from build123d import *

# Parameters (mm, degrees)
CHANFREIN1_SIZE         = 0.2
CONG_1_R                = 0.5
EMPREINTE_POUR_CL_DEPTH = 2.5


with BuildPart() as part:
    # Esquisse1 → Base-Révolution (revolve)
    with BuildSketch(Plane.XY, mode=Mode.PRIVATE) as base_r_volution_sk:
        Polygon((-2.5, 0), (-2.5, 2.25), (0, 2.25), (0, 1.25), (10, 1.25), (10, 0), align=None)
    revolve(base_r_volution_sk.sketch.rotate(Axis((-28.982684825, 0, 0), (1, 0, 0)), 90), axis=Axis((-28.982684825, 0, 0), (1, 0, 0)))

    # Chanfrein1
    chanfrein1_edges = [part.edges().sort_by_distance(p)[0] for p in [
        (10, 0, -1.25),
    ]]
    chamfer(chanfrein1_edges, length=CHANFREIN1_SIZE)

    # Congé1
    cong_1_edges = [part.edges().sort_by_distance(p)[0] for p in [
        (-2.5, 0, -2.25),
    ]]
    fillet(cong_1_edges, radius=CONG_1_R)

    # Esquisse2 → Empreinte pour clé (cut)
    with BuildSketch(Plane.ZY.offset(2.5)):
        Polygon((0.577350269, -1), (-0.577350269, -1), (-1.154700538, 0), (-0.577350269, 1), (0.577350269, 1), (1.154700538, 0), align=None)
    extrude(amount=-EMPREINTE_POUR_CL_DEPTH, mode=Mode.SUBTRACT)


solid = part.part
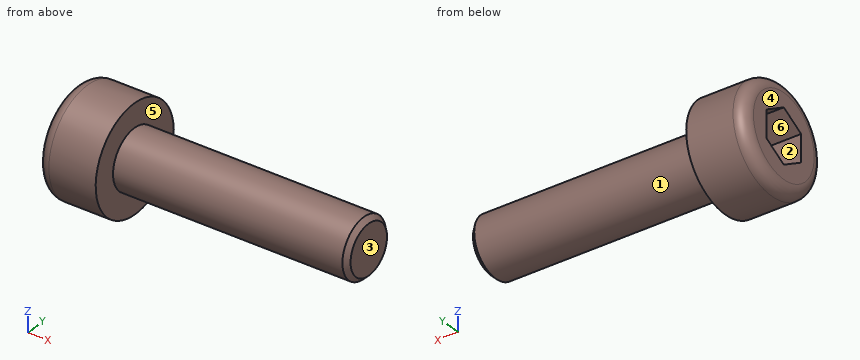
Work out the finished part from the listing and answer in its coordinate system (mm). Face numbers are marked on the shaded views. A direction names the side the tool comes from. Coordinates: 2 decimals unless noted, no trailing zeros. Write each loop counter-clockwise with the first axis right and the second up, starting at its lowest first coordinate (ties: lowest second). Pieces come first, ordered by that corner, then holes. Notation, with made-up numbers: (25.25, 64) - (56.25, 64) arc R30 cw to (56.25, 99) - close; hole circle Ø6 at (-15.75, 81.25). An arc over 180 degrees is marked (long way). One line per question, with ' | ' between items.
1) Consider probe 1 along X at (y, z) = (1, -1.2); probe 2 along X at (y, z) = (-0.05, 0.5); probe 3 along Y at (x, z) = (-0.75, 1.5). Determine where each line is inside the solid, lowest interval first. Write a range as [from, to].
Checks:
probe 1: [-2.5, 0] | probe 2: [0, 10] | probe 3: [-1.68, 1.68]
2) Find section A-A, the plane x = -1.25. Determine the outline of the cut face in (y, z).
Checks:
outline: circle Ø4.5 at (0, 0); hole (-1, -0.58) - (0, -1.15) - (1, -0.58) - (1, 0.58) - (0, 1.15) - (-1, 0.58) - close
3) The mould has two halves that part along Y. Classify the marked faces 1, 2 and 3: +Y half, -Y half, draft (parallel to the pull), parting line (faces both ways), or undercut.
Checks:
face 1: parting line | face 2: undercut | face 3: draft
4) Find section C-C, the plane x = 3.75. Determine the outline of the cut face in (y, z), and give its area (3 significant figures).
Checks:
outline: circle Ø2.5 at (0, 0) | area: 4.91 mm2
5) Find section B-B, the plane z = 0. Determine the outline of the cut face in (x, y).
Checks:
outline: (-2.5, -1.75) arc R0.5 ccw to (-2, -2.25) - (0, -2.25) - (0, -1.25) - (9.8, -1.25) - (10, -1.05) - (10, 1.05) - (9.8, 1.25) - (0, 1.25) - (0, 2.25) - (-2, 2.25) arc R0.5 ccw to (-2.5, 1.75) - (-2.5, 1) - (0, 1) - (0, -1) - (-2.5, -1) - close
6) For the marked faces 4, 5 and 6, determine the directions among +Z, -Z, +X, -X, +Y, -Y from which every point of the face is accessible in a straight line to the end or side of a thin tool.
Checks:
face 4: +Z, -Z, -X, +Y, -Y | face 5: +X | face 6: -X
